Here's the drawing with two shaded views (mm, measured from the low corner). I have some questions. Round coordinates to 2 decimals unless told otherwise and drop trailing zeros. Order: outer loops, then holes, each group sorted by start corner. A loop starts at its lowest first (then second) coordinate and runs counter-clockwise, first axis right, second up. Notation, with made-up numbers: (-6, 29) - (46, 29) arc R32 cw to (46, 64) - close; hole circle Ø1 at (74.25, -1.75). An arc over 180 degrees is marked (long way). Return JSON: item names as keys, results as strings. Group by question number.
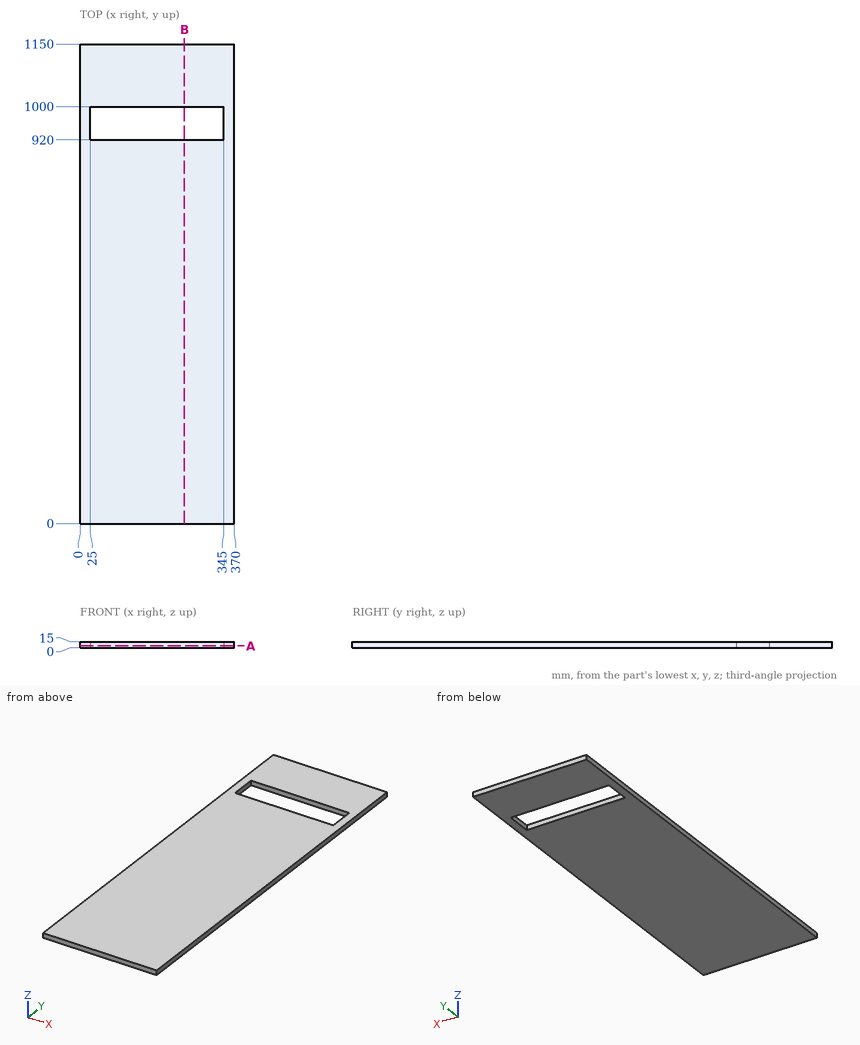
1) If I drill on line 1 along Y through (x, z) = (338, 1.25); line 2 along X through (y, z) = (978, 7.25), over which ranges is the centre line in solid material (lowest first)? Write a range as from..to.
2) Will this pin go through, and if not, where does the flat tip stop? pin 1 (4 mm diameter, centred on x = 66, z = 2.5, fed in from -Y).
3) I want a section at A-A, the plane z = 4.75. List the corners of the cut face in (x, y) for me, plus the area to 3 significant figures.
4) I want a section at B-B, the plane x = 250.5. List the corners of the cut face in (y, z) for me.
Outcome:
{
 "1": {"line 1": "0..920, 1000..1150", "line 2": "0..25, 345..370"},
 "2": {"pin 1": "y = 0"},
 "3": {"outline": "(0, 0) - (370, 0) - (370, 1150) - (0, 1150) - close; hole (25, 920) - (345, 920) - (345, 1000) - (25, 1000) - close", "area": "400,000 mm^2"},
 "4": {"outline": "(0, 0) - (920, 0) - (920, 15) - (0, 15) - close; (1000, 0) - (1150, 0) - (1150, 15) - (1000, 15) - close"}
}
